Geometry check sheet. Reference: the model listing, model coordinates, mm. Give positions to 0.01 mm unless a question says otherwise; leave off trailing zeros. Order: outer loops, then holes, each group sorted by start corner. A loop starts at its lowest first (then second) coordinate and runs counter-clockwise, first axis right, second up. Notation, with made-up numbers: M 3.25,39.5 L 23.25,39.5 A21 cw 23.25,75.5 Z; hole C 12,56 d11. An arc over 180 degrees is marked long. Answer as CSV lines item,"result". Start each with the question number.
```python
from build123d import *

# Parameters (mm, degrees)
SKETCH1_W      = 16
SKETCH1_H      = 16
EXTRUDE1_DEPTH = 208
SKETCH2_W      = 13
SKETCH2_H      = 13
EXTRUDE2_DEPTH = 210.22714929
SKETCH3_R      = 4
SKETCH3_R_2    = 1.85
EXTRUDE3_DEPTH = 210.22714929
SKETCH4_R      = 4
SKETCH4_R_2    = 1.85
EXTRUDE4_DEPTH = 210.22714929
FILLET1_R      = 1


with BuildPart() as part:
    # Sketch1 → Extrude1 (new body)
    with BuildSketch(Plane.XY):
        with Locations((8, 8)):
            Rectangle(SKETCH1_W, SKETCH1_H)
    extrude(amount=-EXTRUDE1_DEPTH)

    # Sketch2 → Extrude2 (cut, through all)
    with BuildSketch(Plane.XY):
        with Locations((8, 8)):
            Rectangle(SKETCH2_W, SKETCH2_H)
    extrude(amount=-EXTRUDE2_DEPTH, mode=Mode.SUBTRACT)

    # Sketch3 → Extrude3 (cut, through all)
    with BuildSketch(Plane(origin=(0, 16, 0), x_dir=(1, 0, 0), z_dir=(0, 1, 0))):
        with Locations(Location((8, 64, 0), (0, 0, 270))):
            Circle(SKETCH3_R)
        with Locations(Location((8, 32, 0), (0, 0, 270))):
            Circle(SKETCH3_R)
        with Locations((8, 0)):
            Circle(SKETCH3_R)
        with Locations(Location((8, 96, 0), (0, 0, 270))):
            Circle(SKETCH3_R)
        with Locations(Location((8, 128, 0), (0, 0, 270))):
            Circle(SKETCH3_R)
        with Locations(Location((8, 160, 0), (0, 0, 270))):
            Circle(SKETCH3_R)
        with Locations(Location((8, 192, 0), (0, 0, 270))):
            Circle(SKETCH3_R)
        with Locations((8, 224)):
            Circle(SKETCH3_R)
        with Locations((8, 256)):
            Circle(SKETCH3_R)
        with Locations(Location((8, 48, 0), (0, 0, 270))):
            Circle(SKETCH3_R)
        with Locations(Location((8, 56, 0), (0, 0, 270))):
            Circle(SKETCH3_R_2)
        with Locations(Location((8, 40, 0), (0, 0, 270))):
            Circle(SKETCH3_R_2)
        with Locations(Location((8, 80, 0), (0, 0, 270))):
            Circle(SKETCH3_R)
        with Locations(Location((8, 88, 0), (0, 0, 270))):
            Circle(SKETCH3_R_2)
        with Locations(Location((8, 72, 0), (0, 0, 270))):
            Circle(SKETCH3_R_2)
        with Locations(Location((8, 16, 0), (0, 0, 270))):
            Circle(SKETCH3_R)
        with Locations(Location((8, 24, 0), (0, 0, 270))):
            Circle(SKETCH3_R_2)
        with Locations(Location((8, 8, 0), (0, 0, 270))):
            Circle(SKETCH3_R_2)
        with Locations(Location((8, 112, 0), (0, 0, 270))):
            Circle(SKETCH3_R)
        with Locations(Location((8, 120, 0), (0, 0, 270))):
            Circle(SKETCH3_R_2)
        with Locations(Location((8, 104, 0), (0, 0, 270))):
            Circle(SKETCH3_R_2)
        with Locations(Location((8, 144, 0), (0, 0, 270))):
            Circle(SKETCH3_R)
        with Locations(Location((8, 152, 0), (0, 0, 270))):
            Circle(SKETCH3_R_2)
        with Locations(Location((8, 136, 0), (0, 0, 270))):
            Circle(SKETCH3_R_2)
        with Locations(Location((8, 176, 0), (0, 0, 270))):
            Circle(SKETCH3_R)
        with Locations(Location((8, 184, 0), (0, 0, 270))):
            Circle(SKETCH3_R_2)
        with Locations(Location((8, 168, 0), (0, 0, 270))):
            Circle(SKETCH3_R_2)
        with Locations((8, 208)):
            Circle(SKETCH3_R)
        with Locations((8, 216)):
            Circle(SKETCH3_R_2)
        with Locations(Location((8, 200, 0), (0, 0, 270))):
            Circle(SKETCH3_R_2)
        with Locations((8, 240)):
            Circle(SKETCH3_R)
        with Locations((8, 248)):
            Circle(SKETCH3_R_2)
        with Locations((8, 232)):
            Circle(SKETCH3_R_2)
    extrude(amount=-EXTRUDE3_DEPTH, mode=Mode.SUBTRACT)

    # Sketch4 → Extrude4 (cut, through all)
    with BuildSketch(Plane(origin=(16, 0, 0), x_dir=(0, 0, -1), z_dir=(1, 0, 0))):
        with Locations(Location((32, 8, 0), (0, 0, 90))):
            Circle(SKETCH4_R)
        with Locations(Location((64, 8, 0), (0, 0, 90))):
            Circle(SKETCH4_R)
        with Locations((0, 8)):
            Circle(SKETCH4_R)
        with Locations(Location((96, 8, 0), (0, 0, 90))):
            Circle(SKETCH4_R)
        with Locations(Location((128, 8, 0), (0, 0, 90))):
            Circle(SKETCH4_R)
        with Locations(Location((160, 8, 0), (0, 0, 90))):
            Circle(SKETCH4_R)
        with Locations(Location((192, 8, 0), (0, 0, 90))):
            Circle(SKETCH4_R)
        with Locations((224, 8)):
            Circle(SKETCH4_R)
        with Locations((256, 8)):
            Circle(SKETCH4_R)
        with Locations(Location((48, 8.074203, 0), (0, 0, 90))):
            Circle(SKETCH4_R)
        with Locations(Location((40, 8.074203, 0), (0, 0, 90))):
            Circle(SKETCH4_R_2)
        with Locations(Location((56, 8.074203, 0), (0, 0, 90))):
            Circle(SKETCH4_R_2)
        with Locations(Location((80, 8, 0), (0, 0, 90))):
            Circle(SKETCH4_R)
        with Locations(Location((72, 8, 0), (0, 0, 90))):
            Circle(SKETCH4_R_2)
        with Locations(Location((88, 8, 0), (0, 0, 90))):
            Circle(SKETCH4_R_2)
        with Locations(Location((16, 8, 0), (0, 0, 90))):
            Circle(SKETCH4_R)
        with Locations(Location((8, 8, 0), (0, 0, 90))):
            Circle(SKETCH4_R_2)
        with Locations(Location((24, 8, 0), (0, 0, 90))):
            Circle(SKETCH4_R_2)
        with Locations(Location((112, 8, 0), (0, 0, 90))):
            Circle(SKETCH4_R)
        with Locations(Location((104, 8, 0), (0, 0, 90))):
            Circle(SKETCH4_R_2)
        with Locations(Location((120, 8, 0), (0, 0, 90))):
            Circle(SKETCH4_R_2)
        with Locations(Location((144, 8, 0), (0, 0, 90))):
            Circle(SKETCH4_R)
        with Locations(Location((136, 8, 0), (0, 0, 90))):
            Circle(SKETCH4_R_2)
        with Locations(Location((152, 8, 0), (0, 0, 90))):
            Circle(SKETCH4_R_2)
        with Locations(Location((176, 8, 0), (0, 0, 90))):
            Circle(SKETCH4_R)
        with Locations(Location((168, 8, 0), (0, 0, 90))):
            Circle(SKETCH4_R_2)
        with Locations(Location((184, 8, 0), (0, 0, 90))):
            Circle(SKETCH4_R_2)
        with Locations((208, 8)):
            Circle(SKETCH4_R)
        with Locations(Location((200, 8, 0), (0, 0, 90))):
            Circle(SKETCH4_R_2)
        with Locations((216, 8)):
            Circle(SKETCH4_R_2)
        with Locations((240, 8)):
            Circle(SKETCH4_R)
        with Locations((232, 8)):
            Circle(SKETCH4_R_2)
        with Locations((248, 8)):
            Circle(SKETCH4_R_2)
    extrude(amount=-EXTRUDE4_DEPTH, mode=Mode.SUBTRACT)

    # Fillet1
    fillet1_edges = [part.edges().sort_by_distance(p)[0] for p in [
        (0, 16, -104),
        (16, 16, -104),
        (16, 0, -104),
        (0, 0, -104),
    ]]
    fillet(fillet1_edges, radius=FILLET1_R)


solid = part.part
```
Item 1: Scan lines: line 1 along X through (y, z) = (2.75, -64.5); line 2 along X through (y, z) = (14.9, -88). Record each from-to range of solid material in increasing order.
Item 2: Section check A-A on z = -200. Record the boundary of the cut face in (x, y), then the cut area to 3 significant figures.
Item 3: Draft check along X on faces 1 (the face through (7.29, 0.76, -198.29)), 2 (the face through (15, 2, -208)). Enter one of: pulls with the +X half, pulls with the -X half, needs draft (parallel to the pull), parting line crosses it, or undercut.
Item 4: Section check B-B on z = -176. Record the boundary of the cut face in (x, y).
Item 5: Depth check by flat-ended pin: pin 1 Ø6 at (y, z) = (8, -8) entering from +X. Enter the tip coordinate at first touch or a pass-through.
Numbers:
1,line 1,"0 to 1.5, 14.5 to 16"
1,line 2,"0 to 6.15, 9.85 to 16"
2,outline,"M 0,1 A1 ccw 1,0 L 6.15,0 L 6.15,1.5 L 1.5,1.5 L 1.5,6.15 L 0,6.15 Z; M 0,9.85 L 1.5,9.85 L 1.5,14.5 L 6.15,14.5 L 6.15,16 L 1,16 A1 ccw 0,15 Z; M 9.85,0 L 15,0 A1 ccw 16,1 L 16,6.15 L 14.5,6.15 L 14.5,1.5 L 9.85,1.5 Z; M 9.85,14.5 L 14.5,14.5 L 14.5,9.85 L 16,9.85 L 16,15 A1 ccw 15,16 L 9.85,16 Z"
2,area,"63.9 mm2"
3,face 1,"undercut"
3,face 2,"needs draft"
4,outline,"M 0,1 A1 ccw 1,0 L 4,0 L 4,1.5 L 1.5,1.5 L 1.5,4 L 0,4 Z; M 0,12 L 1.5,12 L 1.5,14.5 L 4,14.5 L 4,16 L 1,16 A1 ccw 0,15 Z; M 12,0 L 15,0 A1 ccw 16,1 L 16,4 L 14.5,4 L 14.5,1.5 L 12,1.5 Z; M 12,14.5 L 14.5,14.5 L 14.5,12 L 16,12 L 16,15 A1 ccw 15,16 L 12,16 Z"
5,pin 1,"x = 16"
